Autodesk Inventor part; units mm, degrees
ref_plane "YZ Plane" through (0, 0, 0) normal (1, 0, 0) x (0, 1, 0)
ref_plane "XZ Plane" through (0, 0, 0) normal (0, 1, 0) x (-1, 0, 0)
ref_plane "XY Plane" through (0, 0, 0) normal (0, 0, 1) x (1, 0, 0)
sketch "Sketch1" plane through (0, 0, 0) normal (0, 1, 0) x (-1, 0, 0)
  line L0 (-1.778, 6.35) -> (-3.302, 6.35)
  arc A0 (-3.302, 6.35) -> (-3.81, 5.842) centre (-3.302, 5.842) ccw
  line L1 (-3.81, 5.842) -> (-3.81, 4.318)
  arc A1 (-3.81, 4.318) -> (-3.302, 3.81) centre (-3.302, 4.318) ccw
  arc A2 (-3.302, 3.81) -> (-3.81, 3.302) centre (-3.302, 3.302) ccw
  line L2 (-3.81, 3.302) -> (-3.81, 1.778)
  arc A3 (-3.81, 1.778) -> (-3.302, 1.27) centre (-3.302, 1.778) ccw
  arc A4 (-3.302, 1.27) -> (-3.81, 0.762) centre (-3.302, 0.762) ccw
  line L3 (-3.81, 0.762) -> (-3.81, -0.762)
  arc A5 (-3.81, -0.762) -> (-3.302, -1.27) centre (-3.302, -0.762) ccw
  line L4 (-3.302, -1.27) -> (-1.778, -1.27)
  arc A6 (-1.778, -1.27) -> (-1.27, -0.762) centre (-1.778, -0.762) ccw
  arc A7 (-1.27, -0.762) -> (-0.762, -1.27) centre (-0.762, -0.762) ccw
  line L5 (-0.762, -1.27) -> (0.762, -1.27)
  arc A8 (0.762, -1.27) -> (1.27, -0.762) centre (0.762, -0.762) ccw
  line L6 (1.27, -0.762) -> (1.27, 0.762)
  arc A9 (1.27, 0.762) -> (0.762, 1.27) centre (0.762, 0.762) ccw
  arc A10 (0.762, 1.27) -> (1.27, 1.778) centre (0.762, 1.778) ccw
  line L7 (1.27, 1.778) -> (1.27, 3.302)
  arc A11 (1.27, 3.302) -> (0.762, 3.81) centre (0.762, 3.302) ccw
  arc A12 (0.762, 3.81) -> (1.27, 4.318) centre (0.762, 4.318) ccw
  line L8 (1.27, 4.318) -> (1.27, 5.842)
  arc A13 (1.27, 5.842) -> (0.762, 6.35) centre (0.762, 5.842) ccw
  line L9 (0.762, 6.35) -> (-0.762, 6.35)
  arc A14 (-0.762, 6.35) -> (-1.27, 5.842) centre (-0.762, 5.842) ccw
  arc A15 (-1.27, 5.842) -> (-1.778, 6.35) centre (-1.778, 5.842) ccw
  arc A16 (-1.27, 0.762) -> (-1.778, 1.27) centre (-1.778, 0.762) ccw
  arc A17 (-1.778, 1.27) -> (-1.27, 1.778) centre (-1.778, 1.778) ccw
  arc A18 (-1.27, 1.778) -> (-0.762, 1.27) centre (-0.762, 1.778) ccw
  arc A19 (-0.762, 1.27) -> (-1.27, 0.762) centre (-0.762, 0.762) ccw
  arc A20 (-1.27, 3.302) -> (-1.778, 3.81) centre (-1.778, 3.302) ccw
  arc A21 (-1.778, 3.81) -> (-1.27, 4.318) centre (-1.778, 4.318) ccw
  arc A22 (-1.27, 4.318) -> (-0.762, 3.81) centre (-0.762, 4.318) ccw
  arc A23 (-0.762, 3.81) -> (-1.27, 3.302) centre (-0.762, 3.302) ccw
extrude "Extrusion1" add sketch "Sketch1" along normal blind 2.54
sketch "Sketch2" plane through (0, 2.54, 0) normal (0, 1, 0) x (1, 0, 0)
  circle A0 centre (0, 0) radius 0.4445
  line L0 (0.762, 1.27) -> (-0.762, 1.27) construction
  line L1 (-1.27, 0.762) -> (-1.27, -0.762) construction
  circle A1 centre (2.54, 0) radius 0.4445
  circle A2 centre (0, -2.54) radius 0.4445
  circle A3 centre (2.54, -2.54) radius 0.4445
  circle A4 centre (0, -5.08) radius 0.4445
  circle A5 centre (2.54, -5.08) radius 0.4445
  dimension "d2" = 0.889
  dimension "d5" = 2.54
  dimension "d8" = 2.54
extrude "Extrusion2" add sketch "Sketch2" along normal blind 5.842 and the other way blind 5.4356
chamfer "Chamfer1" distance 0.381 angle 45 12 edges at (2.0955, 8.382, 5.08) (-0.4445, 8.382, 5.08) (2.0955, 8.382, 2.54) (-0.4445, 8.382, 2.54) (2.0955, 8.382, 0) (-0.4445, 8.382, 0) (2.0955, -2.8956, 5.08) (2.0955, -2.8956, 2.54) (2.0955, -2.8956, 0) (-0.4445, -2.8956, 0) (-0.4445, -2.8956, 2.54) (-0.4445, -2.8956, 5.08)
properties part number "2x3 header"
Can you work these out from the model? Positions are in its coordinate system, mm. A direction names the side the tool comes from. Coordinates: 2 decimals unless noted, no trailing zeros. Write each loop counter-clockwise with the first axis right and the second up, starting at its lowest first coordinate (ties: lowest second). Pieces come first, ordered by that corner, then holes.
Q1. Please list where these lines run through material, in increasing order: L1, parallel to Z at x = -0.2, y = 3.5; L2, parallel to Y at x = 3.35, z = -0.25; L3, parallel to X at y = -0.75, z = 2.5.
Results found:
L1: z = -0.4 to 0.4, 2.14 to 2.94, 4.68 to 5.48
L2: y = 0 to 2.54
L3: x = -0.44 to 0.44, 2.1 to 2.98
Q2. Imagine slicing it at C-C, the plane x = 3.15. List the corners of the cut face in (y, z) for me.
Results found:
outline: (0, -1.27) - (2.54, -1.27) - (2.54, 6.35) - (0, 6.35) - close
Q3. Which directions (+Z, -Z, +X, -X, +Y, -Y) give clear straight access to the entire face, cutting with the end or side of a thin tool? Please do faces 1 (the face through (0, 1, -1.27)), 2 (the face through (-0.096, -1.24, 0.434)), 3 (the face through (2.48, 5.23, 5.52)).
Results found:
face 1: -Z, +X, -X, +Y, -Y
face 2: -Y
face 3: +Y
Q4. Imagine slicing it at B-B, the plane y = 1.75. Count the separate pieces of the cut face and the enclosed holes in it, plus the area to 3 significant figures.
Results found:
separate pieces: 1
enclosed holes: 2
area: 37.4 mm2
Q5. For P1, Ø2.5, axis at x = 1.5, z = 4, coming from the -Y side; P2, Ø1, axis at x = 1, z = 4.5, coming from the +Y side; P3, Ø1, axis at y = 5.5, z = 2.5, coming from the -X side, each with a flat end and sliding along its axis, tell me the tip position at first contact or that it passes through.
Results found:
P1: stops at y = -2.71
P2: stops at y = 2.54
P3: stops at x = -0.44
Q6. If we mould it in two halves opening along Z, with no side actions, what happens to faces 4 (the face through (-0.06, 5.23, 5.52)), 5 (the face through (-1.27, 1, 0)), 6 (the face through (3, 1, 6.35))? For each: +Z half, -Z half, draft (parallel to the pull), parting line (faces both ways), or undercut.
Results found:
face 4: undercut
face 5: draft
face 6: +Z half
Q7. Imagine slicing it at A-A, the plane y = -0.75. List the corners of the cut face in (x, z) for me.
Results found:
outline: circle Ø0.89 at (0, 0); circle Ø0.89 at (0, 2.54); circle Ø0.89 at (0, 5.08); circle Ø0.89 at (2.54, 0); circle Ø0.89 at (2.54, 2.54); circle Ø0.89 at (2.54, 5.08)
